```python
from build123d import *

# Parameters (mm, degrees)
PAD037_DEPTH      = 46
PAD037_DEPTH_BACK = 3
PAD038_DEPTH      = 3
POCKET016_DEPTH   = 10
SKETCH066_R       = 2.1
POCKET023_DEPTH   = 5


with BuildPart() as tentingleg:
    # Sketch054 → Pad037 (new body, two sides)
    with BuildSketch(Plane.XZ) as pad037_sk:
        Polygon((-55, -1), (-5, -1), (1, -1), (1, -31), (3.9999999999, -31), (3.9999999999, -1), (3.9999999999, 2), (-5, 2), (-55, 2), align=None)
    extrude(amount=PAD037_DEPTH)
    extrude(pad037_sk.sketch, amount=-PAD037_DEPTH_BACK)

    # Sketch055 → Pad038 (join)
    with BuildSketch(Plane.XZ):
        with BuildLine():
            ThreePointArc((8.9999999999, -43.2857142857), (12.8523729567, -41.4730678277), (13.9115498355, -37.3494033264))
            ThreePointArc((28.0891318316, -12.7931109807), (16.4349866323, -22.4354486765), (13.9115498355, -37.3494033264))
            ThreePointArc((28.0891318316, -12.7931109807), (31.130741607, -9.8140046459), (30.7743530093, -5.5714285714))
            ThreePointArc((30.7743530093, -5.5714285714), (21.5714285713, 3.6314958666), (8.9999999999, 7))
            ThreePointArc((8.9999999999, 7), (5.464466094, 5.5355339059), (3.9999999999, 2))
            Line((3.9999999999, 2), (1, -1))
            ThreePointArc((-11.2463328898, -24.0732475684), (-2.2513043788, -14.0608903085), (1, -1))
            ThreePointArc((-11.2463328898, -24.0732475684), (-13.3169087301, -27.0931421371), (-12.7743530095, -30.7142857143))
            ThreePointArc((-12.7743530095, -30.7142857143), (-3.5714285715, -39.9172101523), (8.9999999999, -43.2857142857))
        make_face()
        with BuildLine():
            ThreePointArc((6.8999999999, -28.2857142857), (8.9999999999, -30.3857142857), (11.0999999999, -28.2857142857))
            Line((11.0999999999, -28.2857142857), (11.0999999999, -8))
            ThreePointArc((11.0999999999, -8), (8.9999999999, -5.9), (6.8999999999, -8))
            Line((6.8999999999, -8), (6.8999999999, -28.2857142857))
        make_face(mode=Mode.SUBTRACT)
        with BuildLine():
            ThreePointArc((8.9999999999, -40.3857142857), (11.0999999999, -38.2857142857), (8.9999999999, -36.1857142857))
            ThreePointArc((-6.6255726426, -27.1642857143), (-0.0214285715, -33.7684297854), (8.9999999999, -36.1857142857))
            ThreePointArc((-6.6255726426, -27.1642857143), (-9.4942259906, -26.3956323663), (-10.2628793385, -29.2642857143))
            ThreePointArc((-10.2628793385, -29.2642857143), (-2.1214285715, -37.4057364813), (8.9999999999, -40.3857142857))
        make_face(mode=Mode.SUBTRACT)
        with BuildLine():
            ThreePointArc((8.9999999999, 4.1), (6.8999999999, 2), (8.9999999999, -0.1))
            ThreePointArc((24.6255726425, -9.1214285714), (18.0214285713, -2.5172845003), (8.9999999999, -0.1))
            ThreePointArc((24.6255726425, -9.1214285714), (27.4942259904, -9.8900819194), (28.2628793384, -7.0214285714))
            ThreePointArc((28.2628793384, -7.0214285714), (20.1214285713, 1.1200221956), (8.9999999999, 4.1))
        make_face(mode=Mode.SUBTRACT)
    extrude(amount=-PAD038_DEPTH)

    # Sketch056 → Pocket016 (cut, symmetric)
    with BuildSketch(Plane.XY):
        with BuildLine():
            ThreePointArc((-47.9, -2), (-50, 0.1), (-52.1, -2))
            Line((-52.1, -2), (-52.1, -41))
            ThreePointArc((-52.1, -41), (-50, -43.1), (-47.9, -41))
            Line((-47.9, -41), (-47.9, -2))
        make_face()
        with BuildLine():
            ThreePointArc((-27.9, -2), (-30, 0.1), (-32.1, -2))
            Line((-32.1, -2), (-32.1, -41))
            ThreePointArc((-32.1, -41), (-30, -43.1), (-27.9, -41))
            Line((-27.9, -41), (-27.9, -2))
        make_face()
        with BuildLine():
            ThreePointArc((-7.9, -2), (-10, 0.1), (-12.1, -2))
            Line((-12.1, -2), (-12.1, -41))
            ThreePointArc((-12.1, -41), (-10, -43.1), (-7.9, -41))
            Line((-7.9, -41), (-7.9, -2))
        make_face()
    extrude(amount=POCKET016_DEPTH, both=True, mode=Mode.SUBTRACT)

    # Sketch066 (on Face45 of Pocket016) → Pocket023 (cut)
    with BuildSketch(Plane(origin=(3.9999999999, 0, 0), x_dir=(0, 0, 1), z_dir=(1, 0, 0))):
        with Locations((-26, 41)):
            Circle(SKETCH066_R)
        with Locations((-16, 31)):
            Circle(SKETCH066_R)
        with Locations((-16, 21)):
            Circle(SKETCH066_R)
        with Locations((-16, 41)):
            Circle(SKETCH066_R)
        with Locations((-6, 31)):
            Circle(SKETCH066_R)
        with Locations((-6, 41)):
            Circle(SKETCH066_R)
        with Locations((-26, 31)):
            Circle(SKETCH066_R)
        with Locations((-26, 21)):
            Circle(SKETCH066_R)
        with Locations((-26, 11)):
            Circle(SKETCH066_R)
        with Locations((-16, 11)):
            Circle(SKETCH066_R)
        with Locations((-6, 11)):
            Circle(SKETCH066_R)
        with Locations((-6, 21)):
            Circle(SKETCH066_R)
    extrude(amount=-POCKET023_DEPTH, mode=Mode.SUBTRACT)


with BuildPart() as tentingleg_1:
    # Body012 placement: moved
    add(tentingleg.part.moved(Location((140, 47, 0))))


with BuildPart() as part_mirroring:
    # Part__Mirroring: instance of TentingLeg
    add(tentingleg_1.part.mirror(Plane(origin=(119.6685180664, 0, -14.4371900558), x_dir=(1, 0, 0), z_dir=(0, 1, -1.192e-07))))


solid = part_mirroring.part
```
Source: CAD feature listing. Evaluate the final solid. Frame: model axes, mm. A direction names the side the tool comes from. Round coordinates to 2 decimals unless told otherwise and drop trailing zeros. Loops run counter-clockwise (first coordinate to the right, second up) from the corner with the lowest first, then second, coordinate; pieces in that order, holes last. Notation, with made-up numbers: M 27.5,88 L 34.5,88 A21 cw 34.5,97 Z; hole C -36.75,73.25 d11. An arc over 180 degrees is marked long. Use a Markdown table: item, result. Add a question column.
1. Mould query, pull axis Y, two halves, no side actions, for faces 6 (the cylindrical face through (142.521, -17.863, -5.031)), 7 (the cylindrical face through (142.521, -7.278, -7.666)), 8 (the flat face through (142, -24, -31)), 9 (the flat face through (146, -47, -20)). Classes: pulls with the +Y half, pulls with the -Y half, needs draft (parallel to the pull), parting line crosses it, or undercut.
2. Section query C-C on z = 1. Give the number of separate pieces and of enclosed holes in the cut face, then the cut area to 3 significant figures.
3. Section query D-D on x = 115.5. Return the cut outline in (y, z), then the cut area to 3 significant figures.
4. Section query A-A on x = 90. Return the cut outline in (y, z), then the cut area to 3 significant figures.
5. Contact query for flat-ended pins moving along their axis: P1, Ø6.5, axis at y = -16, z = -16, coming from the -X side; P2, Ø1.5, axis at y = -48, z = -16.5, coming from the -X side; P3, Ø14.5, axis at x = 109, y = -37.5, coming from the +Z side; P4, Ø12, axis at x = 145, z = -4, coming from the +Y side. Output: stop coordinate, or through.
6. Line query: line 1 (Z direction, x = 134.5, y = -19.5); line 2 (Z direction, x = 141.5, y = -27.5); line 3 (X direction, y = -39.5, z = -16). Output: solid intervals per line, ascending.
7. Section query B-B on y = -22.5. Return the cut outline in (x, z).
8. Reachability of faces 1 (the flat face through (141, -23.7, -15.8)), 2 (the flat face through (144, -23.7, -14.7)), 3 (the cylindrical face through (158.136, -48.479, -2.584)), 4 (the cylindrical face through (137.66, -48.48, -14.23)), 5 (the flat face through (107.9, -26, 0)) from +Z, -Z, +X, -X, +Y, -Y: full face, straight path, thin tool, end or side. Return the list, or none.
Reported:
| question | item | result |
|---|---|---|
| 1 | face 6 | undercut |
| 1 | face 7 | undercut |
| 1 | face 8 | needs draft |
| 1 | face 9 | pulls with the +Y half |
| 2 | separate pieces | 2 |
| 2 | enclosed holes | 3 |
| 2 | area | 2,380 mm² |
| 3 | outline | M -50,-1 L -1,-1 L -1,2 L -50,2 Z |
| 3 | area | 147 mm² |
| 4 | outline | M -50,-1 L -47.1,-1 L -47.1,2 L -50,2 Z; M -3.9,-1 L -1,-1 L -1,2 L -3.9,2 Z |
| 4 | area | 17.4 mm² |
| 5 | P1 | stops at x = 141 |
| 5 | P2 | stops at x = 135.77 |
| 5 | P3 | stops at z = 2 |
| 5 | P4 | stops at y = -1 |
| 6 | line 1 | z = -1 to 2 |
| 6 | line 2 | z = -31 to -27.47, -24.53 to -17.47, -14.53 to -7.47, -4.53 to 2 |
| 6 | line 3 | x = 141 to 144 |
| 7 | outline | M 85,-1 L 87.9,-1 L 87.9,2 L 85,2 Z; M 92.1,-1 L 107.9,-1 L 107.9,2 L 92.1,2 Z; M 112.1,-1 L 127.9,-1 L 127.9,2 L 112.1,2 Z; M 132.1,-1 L 141,-1 L 141,-31 L 144,-31 L 144,2 L 132.1,2 Z |
| 8 | face 1 | -Z, -X, +Y |
| 8 | face 2 | +Z, -Z, +X, +Y |
| 8 | face 3 | +Y, -Y |
| 8 | face 4 | -X, +Y, -Y |
| 8 | face 5 | +Z, -Z |
